The model under review builds one solid part; all positions refer to its coordinate system, in mm. A direction names the side the tool comes from. Give positions to 0.01 mm unless a question says otherwise; leave off trailing zeros. Write each loop counter-clockwise with the first axis right and the second up, starting at its lowest first coordinate (ties: lowest second). Pieces come first, ordered by that corner, then holes.
from build123d import *

# Parameters (mm, degrees)
SKETCH1_W                                 = 178.5366
SKETCH1_H                                 = 12.7
BOSS_EXTRUDE1_DEPTH                       = 342.9
CUT_EXTRUDE1_REACH                        = 14.7
SKETCH2_W                                 = 127.7366
SKETCH2_H                                 = 292.1
FILLET1_R                                 = 50.8
F_15_64_0_23438_DIAMETER_HOLE2_D          = 5.953252
F_15_64_0_23438_DIAMETER_HOLE2_DEPTH      = 12.7
F_15_64_0_23438_DIAMETER_HOLE2_TIP        = 1.788537341
F_5_64_0_07813_DIAMETER_HOLE1_D           = 1.984502
F_5_64_0_07813_DIAMETER_HOLE1_DEPTH       = 38.1
F_5_64_0_07813_DIAMETER_HOLE1_CSINK_D     = 10.16
F_5_64_0_07813_DIAMETER_HOLE1_CSINK_ANGLE = 82
F_5_64_0_07813_DIAMETER_HOLE1_TIP         = 0.59620455
F_5_64_0_07813_DIAMETER_HOLE2_AT_2_COUNT  = 2
F_5_64_0_07813_DIAMETER_HOLE2_AT_2_PITCH  = 36.5125
F_5_64_0_07813_DIAMETER_HOLE2_AT_3_COUNT  = 2
F_5_64_0_07813_DIAMETER_HOLE2_AT_3_PITCH  = 73.025
F_5_64_0_07813_DIAMETER_HOLE2_AT_4_COUNT  = 2
F_5_64_0_07813_DIAMETER_HOLE2_AT_4_PITCH  = 109.5375
F_5_64_0_07813_DIAMETER_HOLE2_AT_5_COUNT  = 2
F_5_64_0_07813_DIAMETER_HOLE2_AT_5_PITCH  = 146.05
F_5_64_0_07813_DIAMETER_HOLE2_AT_6_COUNT  = 2
F_5_64_0_07813_DIAMETER_HOLE2_AT_6_PITCH  = 182.5625
F_5_64_0_07813_DIAMETER_HOLE2_AT_7_COUNT  = 2
F_5_64_0_07813_DIAMETER_HOLE2_AT_7_PITCH  = 219.075
CUT_EXTRUDE2_REACH                        = 14.7
SKETCH11_W                                = 178.5366
SKETCH11_H                                = 44.45
CUT_EXTRUDE3_START                        = -12.7
SKETCH12_W                                = 127.7366
SKETCH12_H                                = 31.75
CUT_EXTRUDE3_DEPTH                        = 12.7
F_8_CLEARANCE_HOLE1_D                     = 4.9149


with BuildPart() as part:
    # Sketch1 → Boss-Extrude1 (new body)
    with BuildSketch(Plane.XY):
        with Locations((-182.40375, -186.69)):
            Rectangle(SKETCH1_W, SKETCH1_H)
    extrude(amount=BOSS_EXTRUDE1_DEPTH)

    # Sketch2 → Cut-Extrude1 (cut, up to next)
    with BuildSketch(Plane.XZ.offset(193.04), mode=Mode.PRIVATE) as cut_extrude1_sk1:
        with Locations((-182.40375, 171.45)):
            Rectangle(SKETCH2_W, SKETCH2_H)
    cut_extrude1_tool1 = extrude(cut_extrude1_sk1.sketch, amount=-CUT_EXTRUDE1_REACH, mode=Mode.PRIVATE) & part.part
    add(cut_extrude1_tool1.solids().sort_by_distance((-182.40375, -193.04, 171.45))[0], mode=Mode.SUBTRACT)

    # Fillet1
    fillet1_edges = [part.edges().sort_by_distance(p)[0] for p in [
        (-118.53545, -186.69, 317.5),
        (-118.53545, -186.69, 25.4),
        (-246.27205, -186.69, 25.4),
        (-246.27205, -186.69, 317.5),
    ]]
    fillet(fillet1_edges, radius=FILLET1_R)

    # 15/64 (0.23438) Diameter Hole2
    with Locations(Plane(origin=(-182.40375, 1936.853954382, -6.35), x_dir=(1, 0, 0), z_dir=(0, 0, -1))):
        with Locations((-262.8265, 2051.088542934), (-262.8265, 2014.068680083), (-262.8265, 1977.048817232), (-98.7933, 2115.959791125), (-98.7933, 2151.166454382), (-44.63415, 2123.543954382), (0, 2123.543954382), (44.63415, 2123.543954382)):
            Hole(F_15_64_0_23438_DIAMETER_HOLE2_D / 2, depth=F_15_64_0_23438_DIAMETER_HOLE2_DEPTH)
            with Locations((0, 0, -(F_15_64_0_23438_DIAMETER_HOLE2_DEPTH + F_15_64_0_23438_DIAMETER_HOLE2_TIP / 2))):  # 118° drill point
                Cone(0, F_15_64_0_23438_DIAMETER_HOLE2_D / 2, F_15_64_0_23438_DIAMETER_HOLE2_TIP, mode=Mode.SUBTRACT)

    # 5/64 (0.07813) Diameter Hole1
    with Locations(Plane(origin=(-182.40375, 1936.853954382, 361.95), x_dir=(-1, 0, 0), z_dir=(0, 0, 1))):
        with Locations((-262.508471454, 2038.114708605), (262.8265, 2038.74858865), (262.8265, 1989.388771516), (262.8265, 1964.708862949), (262.8265, 2014.068680083), (262.8265, 2063.428497217), (98.7933, 2131.851871048), (98.7933, 2093.487287715), (98.7933, 2055.122704382), (98.7933, 2016.758121048), (98.7933, 1978.393537715), (53.56098, 2123.543954382), (-53.56098, 2123.543954382), (-98.330098001, 1978.155684545), (-98.422680867, 2016.520156166), (-98.515263732, 2054.884627786), (-98.607846597, 2093.249099407), (-98.700429462, 2131.613571028), (-262.568029943, 2062.794545307), (-262.448912964, 2013.434871902), (-262.329795984, 1964.075198497), (-262.389354474, 1988.755035199)):
            CounterSinkHole(F_5_64_0_07813_DIAMETER_HOLE1_D / 2, F_5_64_0_07813_DIAMETER_HOLE1_CSINK_D / 2, depth=F_5_64_0_07813_DIAMETER_HOLE1_DEPTH, counter_sink_angle=F_5_64_0_07813_DIAMETER_HOLE1_CSINK_ANGLE)
            with Locations((0, 0, -(F_5_64_0_07813_DIAMETER_HOLE1_DEPTH + F_5_64_0_07813_DIAMETER_HOLE1_TIP / 2))):  # 118° drill point
                Cone(0, F_5_64_0_07813_DIAMETER_HOLE1_D / 2, F_5_64_0_07813_DIAMETER_HOLE1_TIP, mode=Mode.SUBTRACT)

    # Sketch10 → 5/64 (0.07813) Diameter Hole2 (revolve, cut)
    with BuildSketch(Plane(origin=(-271.67205, -186.69, 280.9875), x_dir=(0, 0, 1), z_dir=(0, 1, 0))):
        Polygon((0, 0), (0, 19.64620455), (0.992251, 19.05), (0.992251, 0), align=None)
    f_5_64_0_07813_diameter_hole2 = revolve(axis=Axis((-278.02205, -186.69, 280.9875), (1, 0, 0)), mode=Mode.SUBTRACT)

    # 5/64 (0.07813) Diameter Hole2 at 2: 5/64 (0.07813) Diameter Hole2 ×2
    with Locations(*[(0, 0, -i * F_5_64_0_07813_DIAMETER_HOLE2_AT_2_PITCH) for i in range(1, F_5_64_0_07813_DIAMETER_HOLE2_AT_2_COUNT)]):
        add(f_5_64_0_07813_diameter_hole2, mode=Mode.SUBTRACT)

    # 5/64 (0.07813) Diameter Hole2 at 3: 5/64 (0.07813) Diameter Hole2 ×2
    with Locations(*[(0, 0, -i * F_5_64_0_07813_DIAMETER_HOLE2_AT_3_PITCH) for i in range(1, F_5_64_0_07813_DIAMETER_HOLE2_AT_3_COUNT)]):
        add(f_5_64_0_07813_diameter_hole2, mode=Mode.SUBTRACT)

    # 5/64 (0.07813) Diameter Hole2 at 4: 5/64 (0.07813) Diameter Hole2 ×2
    with Locations(*[(0, 0, -i * F_5_64_0_07813_DIAMETER_HOLE2_AT_4_PITCH) for i in range(1, F_5_64_0_07813_DIAMETER_HOLE2_AT_4_COUNT)]):
        add(f_5_64_0_07813_diameter_hole2, mode=Mode.SUBTRACT)

    # 5/64 (0.07813) Diameter Hole2 at 5: 5/64 (0.07813) Diameter Hole2 ×2
    with Locations(*[(0, 0, -i * F_5_64_0_07813_DIAMETER_HOLE2_AT_5_PITCH) for i in range(1, F_5_64_0_07813_DIAMETER_HOLE2_AT_5_COUNT)]):
        add(f_5_64_0_07813_diameter_hole2, mode=Mode.SUBTRACT)

    # 5/64 (0.07813) Diameter Hole2 at 6: 5/64 (0.07813) Diameter Hole2 ×2
    with Locations(*[(0, 0, -i * F_5_64_0_07813_DIAMETER_HOLE2_AT_6_PITCH) for i in range(1, F_5_64_0_07813_DIAMETER_HOLE2_AT_6_COUNT)]):
        add(f_5_64_0_07813_diameter_hole2, mode=Mode.SUBTRACT)

    # 5/64 (0.07813) Diameter Hole2 at 7: 5/64 (0.07813) Diameter Hole2 ×2
    with Locations(*[(0, 0, -i * F_5_64_0_07813_DIAMETER_HOLE2_AT_7_PITCH) for i in range(1, F_5_64_0_07813_DIAMETER_HOLE2_AT_7_COUNT)]):
        add(f_5_64_0_07813_diameter_hole2, mode=Mode.SUBTRACT)

    # Mirror1: 5/64 (0.07813) Diameter Hole2 across plane
    add(f_5_64_0_07813_diameter_hole2.mirror(Plane.ZY.offset(182.40375)), mode=Mode.SUBTRACT)

    # Mirror1 copy 1 sketch → Mirror1 copy 1 (revolve, cut)
    with BuildSketch(Plane(origin=(-93.13545, -186.69, 244.475), x_dir=(0, 0, 1), z_dir=(0, 1, 0))):
        Polygon((0, 0), (0, -19.64620455), (0.992251, -19.05), (0.992251, 0), align=None)
    revolve(axis=Axis((-86.78545, -186.69, 244.475), (1, 0, 0)), mode=Mode.SUBTRACT)

    # Mirror1 copy 2 sketch → Mirror1 copy 2 (revolve, cut)
    with BuildSketch(Plane(origin=(-93.13545, -186.69, 207.9625), x_dir=(0, 0, 1), z_dir=(0, 1, 0))):
        Polygon((0, 0), (0, -19.64620455), (0.992251, -19.05), (0.992251, 0), align=None)
    revolve(axis=Axis((-86.78545, -186.69, 207.9625), (1, 0, 0)), mode=Mode.SUBTRACT)

    # Mirror1 copy 3 sketch → Mirror1 copy 3 (revolve, cut)
    with BuildSketch(Plane(origin=(-93.13545, -186.69, 171.45), x_dir=(0, 0, 1), z_dir=(0, 1, 0))):
        Polygon((0, 0), (0, -19.64620455), (0.992251, -19.05), (0.992251, 0), align=None)
    revolve(axis=Axis((-86.78545, -186.69, 171.45), (1, 0, 0)), mode=Mode.SUBTRACT)

    # Mirror1 copy 4 sketch → Mirror1 copy 4 (revolve, cut)
    with BuildSketch(Plane(origin=(-93.13545, -186.69, 134.9375), x_dir=(0, 0, 1), z_dir=(0, 1, 0))):
        Polygon((0, 0), (0, -19.64620455), (0.992251, -19.05), (0.992251, 0), align=None)
    revolve(axis=Axis((-86.78545, -186.69, 134.9375), (1, 0, 0)), mode=Mode.SUBTRACT)

    # Mirror1 copy 5 sketch → Mirror1 copy 5 (revolve, cut)
    with BuildSketch(Plane(origin=(-93.13545, -186.69, 98.425), x_dir=(0, 0, 1), z_dir=(0, 1, 0))):
        Polygon((0, 0), (0, -19.64620455), (0.992251, -19.05), (0.992251, 0), align=None)
    revolve(axis=Axis((-86.78545, -186.69, 98.425), (1, 0, 0)), mode=Mode.SUBTRACT)

    # Mirror1 copy 6 sketch → Mirror1 copy 6 (revolve, cut)
    with BuildSketch(Plane(origin=(-93.13545, -186.69, 61.9125), x_dir=(0, 0, 1), z_dir=(0, 1, 0))):
        Polygon((0, 0), (0, -19.64620455), (0.992251, -19.05), (0.992251, 0), align=None)
    revolve(axis=Axis((-86.78545, -186.69, 61.9125), (1, 0, 0)), mode=Mode.SUBTRACT)

    # Sketch11 → Cut-Extrude2 (cut, up to next)
    with BuildSketch(Plane.XZ.offset(193.04), mode=Mode.PRIVATE) as cut_extrude2_sk1:
        with Locations((-182.40375, 22.225)):
            Rectangle(SKETCH11_W, SKETCH11_H)
    cut_extrude2_tool1 = extrude(cut_extrude2_sk1.sketch, amount=-CUT_EXTRUDE2_REACH, mode=Mode.PRIVATE) & part.part
    add(cut_extrude2_tool1.solids().sort_by_distance((-182.40375, -193.04, 22.225))[0], mode=Mode.SUBTRACT)

    # Sketch12 → Cut-Extrude3 (cut)
    with BuildSketch(Plane.XZ.offset(193.04).offset(CUT_EXTRUDE3_START)):
        with Locations((-182.40375, 60.325)):
            Rectangle(SKETCH12_W, SKETCH12_H)
    extrude(amount=CUT_EXTRUDE3_DEPTH, mode=Mode.SUBTRACT)

    # #8 Clearance Hole1 (through all)
    with Locations(Plane(origin=(0, -193.04, 0), x_dir=(-1, 0, 0), z_dir=(0, -1, 0))):
        with Locations((261.3533, -85.725), (261.3533, -57.15), (103.4542, -57.15), (103.4542, -85.725)):
            Hole(F_8_CLEARANCE_HOLE1_D / 2)


solid = part.part
1) The part is to be moulded in two halves that separate along X. For faces 1 (the flat face through (-259, -187, 44.45)), 2 (the flat face through (-271.672, -187, 192)), 3 (the cylindrical face through (-231.79, -186.6, 302.22)), say which applies: +X half, -X half, draft (parallel to the pull), parting line (faces both ways), or undercut.
2) Insertion check: pin 1 (1.6 mm diameter, centred on y = -186.69, z = 134.94, fed in from -X); pin 2 (3 mm diameter, centred on y = -186.69, z = 61.91, fed in from +X); pin 3 (1.8 mm diameter, centred on y = -186.69, z = 244.475, fed in from +X); pin 4 (1 mm diameter, centred on x = -226.5, y = -188, fed in from -Z). Each pin has a flat end and moves straight along its axis. Give the tip position at first contact, or say it passes through.
3) Tool access review of faces 4 (the flat face through (-246.272, -187, 154)), 5 (the flat face through (-117, -180.34, 226)): name each direction out of +Z, -Z, +X, -X, +Y, -Y from which nothing blocks a thin tool from reaching the whole face with its end or side.
4) To check wall thickness, follow probe 1 along X at (y, z) = (-185.25, 57.15); probe 2 along X at (y, z) = (-188.5, 125); probe 3 along Z at (x, y) = (-101.5, -182). State the ranges of each line that lie inside material, in increasing order.
5) Consider section A-A, the plane z = 73. Give the boundary of the cut face in (x, y).
6) Consider section B-B, the plane y = -190.25. Give the boundary of the cut face in (x, z) (3 decimals).
7) Consider section D-D, the plane x = -150.5. Give the boundary of the cut face in (y, z).
8) Consider section C-C, the plane x = -181. Give the boundary of the cut face in (y, z), then the cut area to 3 significant figures.
Answer block:
1. face 1: draft
1. face 2: -X half
1. face 3: undercut
2. pin 1: stops at x = -252.51
2. pin 2: stops at x = -93.14
2. pin 3: stops at x = -112.24
2. pin 4: stops at z = 306.53
3. face 4: -Z, +Y, -Y
3. face 5: +Z, -Z, +X, -X, +Y
4. probe 1: x = -271.67 to -263.81, -258.9 to -246.27, -118.54 to -105.91, -101 to -93.14
4. probe 2: x = -271.67 to -246.27, -118.54 to -93.14
4. probe 3: z = 44.45 to 55.66, 58.64 to 84.23, 87.22 to 342.9
5. outline: (-271.67, -193.04) - (-246.27, -193.04) - (-246.27, -180.34) - (-271.67, -180.34) - close; (-118.54, -193.04) - (-93.14, -193.04) - (-93.14, -180.34) - (-118.54, -180.34) - close
6. outline: (-271.672, 44.45) - (-246.272, 44.45) - (-246.272, 266.7) arc R50.8 cw to (-195.472, 317.5) - (-169.335, 317.5) arc R50.8 cw to (-118.535, 266.7) - (-118.535, 44.45) - (-93.135, 44.45) - (-93.135, 342.9) - (-271.672, 342.9) - close; hole circle Ø4.915 at (-261.353, 57.15); hole circle Ø4.915 at (-261.353, 85.725); hole circle Ø4.915 at (-103.454, 57.15); hole circle Ø4.915 at (-103.454, 85.725)
7. outline: (-193.04, 313.88) - (-180.34, 313.88) - (-180.34, 342.9) - (-193.04, 342.9) - close
8. outline: (-193.04, 317.5) - (-180.34, 317.5) - (-180.34, 342.9) - (-193.04, 342.9) - close
8. area: 323 mm2
